Part model, mm, in its own coordinate system. A direction names the side the tool comes from. Round coordinates to 2 decimals unless told otherwise and drop trailing zeros. Order: outer loops, then holes, each group sorted by start corner. A loop starts at its lowest first (then second) coordinate and runs counter-clockwise, first axis right, second up. Notation, with made-up numbers: (74.25, 9) -> (122.25, 9) arc R20 ccw to (122.25, 27) -> close; hole circle Ø1 at (80.5, 70.5). An arc over 180 degrees is marked (long way). Use CSV: the item, a comma, the result in double quotes.
```python
from build123d import *

# Parameters (mm, degrees)
F0_W     = 25.4
F0_H     = 25.4
F1_DEPTH = 17.78
F0_H_2   = 91.44
F2_DEPTH = 68.58
F3_W     = 50.8
F3_H     = 25.4
F3_H_2   = 40.64
F4_DEPTH = 17.78
F5_W     = 25.4
F5_H     = 25.4
F6_DEPTH = 25.4
F7_W     = 25.4
F7_H     = 25.4
F7_H_2   = 40.64
F8_DEPTH = 25.4


with BuildPart() as f1:
    # F0 (on Front) → F1 (new body)
    with BuildSketch(Plane.XZ):
        with Locations((45.547863, 42.605166)):
            Rectangle(F0_W, F0_H)
    extrude(amount=F1_DEPTH)

    # F0 (on Front) → F2 (join)
    with BuildSketch(Plane.XZ):
        with Locations((45.547863, -15.814834)):
            Rectangle(F0_W, F0_H_2)
    extrude(amount=F2_DEPTH)

    # F3 (on face) → F4 (join)
    with BuildSketch(Plane.YZ.offset(58.247863)):
        with Locations((-43.18, -48.834834)):
            Rectangle(F3_W, F3_H)
        with Locations((-43.18, 9.585166)):
            Rectangle(F3_W, F3_H_2)
    extrude(amount=F4_DEPTH)

    # F5 (on face) → F6 (cut)
    with BuildSketch(Plane.XZ.offset(68.58)):
        with Locations((45.547863, -23.434834)):
            Rectangle(F5_W, F5_H)
    extrude(amount=-F6_DEPTH, mode=Mode.SUBTRACT)

    # F7 (on face) → F8 (join)
    with BuildSketch(Plane(origin=(32.847863, 0, 0), x_dir=(0, -1, 0), z_dir=(-1, 0, 0))):
        with Locations((55.88, -48.834834)):
            Rectangle(F7_W, F7_H)
        with Locations((55.88, 9.585166)):
            Rectangle(F7_W, F7_H_2)
    extrude(amount=F8_DEPTH)


solid = f1.part
```
(1) Probe probe 1 along Z at (x, y) = (68.5, -60); probe 2 along Y at (x, z) = (51, 48); probe 3 along X at (y, z) = (-26.5, 14). List the from-to ranges inside material, lowest first. Write a range as [from, to].
Reply:
probe 1,"[-61.53, -36.13], [-10.73, 29.91]"
probe 2,"[-17.78, 0]"
probe 3,"[32.85, 76.03]"
(2) Drop flat-ended pins along their axis: P1, Ø2, axis at y = -9, z = 10, coming from the -X side; P2, Ø20.5, axis at x = 20.5, z = 2.5, coming from the +Y side; P3, Ø1, axis at x = 58.5, z = 12.5, coming from the +Y side; P4, Ø4, axis at y = -15.5, z = -34, coming from the +X side. Give the stop position or say it passes through.
Reply:
P1,"x = 32.85"
P2,"y = -43.18"
P3,"y = 0"
P4,"x = 58.25"
(3) Cut at D-D, the plane x = 52.5. Give the cut face in (y, z).
Reply:
outline,"(-68.58, -61.53) -> (0, -61.53) -> (0, 55.31) -> (-17.78, 55.31) -> (-17.78, 29.91) -> (-68.58, 29.91) -> (-68.58, -10.73) -> (-43.18, -10.73) -> (-43.18, -36.13) -> (-68.58, -36.13) -> close"
(4) Cut at A-A, the plane x = 67.5. Give the cut face in (y, z).
Reply:
outline,"(-68.58, -61.53) -> (-17.78, -61.53) -> (-17.78, -36.13) -> (-68.58, -36.13) -> close; (-68.58, -10.73) -> (-17.78, -10.73) -> (-17.78, 29.91) -> (-68.58, 29.91) -> close"
(5) Cut at B-B, the plane y = -48. Give the cut face in (x, z), then the cut area to 3 significant figures.
Reply:
outline,"(7.45, -61.53) -> (76.03, -61.53) -> (76.03, -36.13) -> (7.45, -36.13) -> close; (7.45, -10.73) -> (76.03, -10.73) -> (76.03, 29.91) -> (7.45, 29.91) -> close"
area,"4,530 mm2"
(6) Pull direction Z, two halves, no side cores. Call faces 5 (the face through (50, -54, -36.135)), 6 (the face through (45, -17.78, 43)), 7 (the face through (45, -9, 55.305)), 8 (the face through (58.248, -12, -4)): released by +Z, released by -Z, zero draft, split by the parting line, or undercut.
Reply:
face 5,"undercut"
face 6,"zero draft"
face 7,"released by +Z"
face 8,"undercut"
(7) Which spindle directions (+Z, -Z, +X, -X, +Y, -Y) get a long thin tool onto all of the face, cutting with end or side? Do faces 1 (the face through (20, -43.18, 9)), 2 (the face through (67, -17.78, 9)), 3 (the face through (49, -43, 29.905)), 4 (the face through (50, -54, -10.735)). Say none if no direction does.
Reply:
face 1,"+Z, -Z, -X, +Y"
face 2,"+Z, -Z, +X, +Y"
face 3,"+Z, +X, -X, -Y"
face 4,"+X, -Y"
(8) Cut at C-C, the plane z = 25.5. Give the cut face in (x, y).
Reply:
outline,"(7.45, -68.58) -> (76.03, -68.58) -> (76.03, -17.78) -> (58.25, -17.78) -> (58.25, 0) -> (32.85, 0) -> (32.85, -43.18) -> (7.45, -43.18) -> close"
